from build123d import *

# Parameters (mm, degrees)
BOSS_EXTRUDE1_DEPTH = 0.11
CUT_EXTRUDE1_DEPTH  = 62.727320532
BOSS_EXTRUDE2_START = -0.11
BOSS_EXTRUDE2_DEPTH = 0.11


with BuildPart() as part:
    # Sketch3 → Boss-Extrude1 (new body)
    with BuildSketch(Plane.XY):
        with BuildLine():
            Line((-12.5, 60), (4.5, 60))
            ThreePointArc((4.5, 60), (11.571067812, 57.071067812), (14.5, 50))
            Line((14.5, 50), (14.5, -58))
            ThreePointArc((14.5, -58), (13.914213562, -59.414213562), (12.5, -60))
            Line((12.5, -60), (-12.5, -60))
            ThreePointArc((-12.5, -60), (-13.914213562, -59.414213562), (-14.5, -58))
            Line((-14.5, -58), (-14.5, 58))
            ThreePointArc((-14.5, 58), (-13.914213562, 59.414213562), (-12.5, 60))
        make_face()
    extrude(amount=BOSS_EXTRUDE1_DEPTH)

    # Sketch4 → Cut-Extrude1 (cut, through all)
    with BuildSketch(Plane.XY.offset(0.11)):
        with BuildLine():
            Line((-14.5, -23), (14.5, -23))
            Line((14.5, -23), (14.5, 50))
            ThreePointArc((14.5, 50), (11.571067812, 57.071067812), (4.5, 60))
            Line((4.5, 60), (-12.5, 60))
            ThreePointArc((-12.5, 60), (-13.914213562, 59.414213562), (-14.5, 58))
            Line((-14.5, 58), (-14.5, -23))
        make_face()
    extrude(amount=-CUT_EXTRUDE1_DEPTH, mode=Mode.SUBTRACT)

    # Sketch5 → Boss-Extrude2 (add)
    with BuildSketch(Plane.XY.offset(0.11).offset(BOSS_EXTRUDE2_START)):
        with BuildLine():
            Line((14.5, -63), (14.5, -23))
            Line((14.5, -23), (-14.5, -23))
            Line((-14.5, -23), (-14.5, -58))
            ThreePointArc((-14.5, -58), (-13.914213562, -59.414213562), (-12.5, -60))
            Line((-12.5, -60), (-3.828427125, -60))
            ThreePointArc((-3.828427125, -60), (-3.06306026, -60.152240935), (-2.414213562, -60.585786438))
            Line((-2.414213562, -60.585786438), (1.414213562, -64.414213562))
            ThreePointArc((1.414213562, -64.414213562), (2.06306026, -64.847759065), (2.828427125, -65))
            Line((2.828427125, -65), (12.5, -65))
            ThreePointArc((12.5, -65), (13.914213562, -64.414213562), (14.5, -63))
        make_face()
    extrude(amount=BOSS_EXTRUDE2_DEPTH)


solid = part.part
Verification items for the finished model (mm, model axes). Give positions to 0.01 mm unless a question says otherwise; leave off trailing zeros. Write each loop counter-clockwise with the first axis right and the second up, starting at its lowest first coordinate (ties: lowest second). Pieces come first, ordered by that corner, then holes. Notation, with made-up numbers: M -25,41.25 L -12,41.25 A22 cw -12,51.25 Z; hole C 20,55 d4. An arc over 180 degrees is marked long. Put each result on its own line as item: value. Start each with the question number.
1. Section check B-B (x = -5.75). Record the cut outline in (y, z).
2. Scan lines: line 1 along Y through (x, z) = (-7.75, 0.05); line 2 along Y through (x, z) = (0, 0.05). Record each from-to range of solid material in increasing order. Write a range as [from, to].
3. Section check A-A (z = 0.05). Record the cut outline in (x, y), and give its area (3 significant figures).
4. Section check C-C (x = -1.25). Record the cut outline in (y, z).
Answer list:
1. outline: M -60,0 L -23,0 L -23,0.11 L -60,0.11 Z
2. line 1: [-60, -23]
2. line 2: [-63, -23]
3. outline: M -14.5,-58 A2 ccw -12.5,-60 L -3.83,-60 A2 cw -2.41,-60.59 L 1.41,-64.41 A2 ccw 2.83,-65 L 12.5,-65 A2 ccw 14.5,-63 L 14.5,-23 L -14.5,-23 Z
3. area: 1,150 mm2
4. outline: M -61.75,0 L -23,0 L -23,0.11 L -61.75,0.11 Z
